from build123d import *

# Parameters (mm, degrees)
PAD048_DEPTH    = 20
PAD049_DEPTH    = 3
CHAMFER030_SIZE = 2
CHAMFER031_SIZE = 1
SKETCH091_R     = 1.6
POCKET029_DEPTH = 5
CHAMFER032_SIZE = 1
SKETCH092_R     = 1.6
POCKET030_DEPTH = 3
CHAMFER033_SIZE = 1
SKETCH093_R     = 1.6
POCKET031_DEPTH = 3.001
CHAMFER034_SIZE = 1


with BuildPart() as part:
    # Sketch089 → Pad048 (new body)
    with BuildSketch(Plane.XY):
        Polygon((19.414214, 3), (8.313708, 3), (3, 8.313708), (3, 19.414214), (1, 21.414214), (0, 21.414214), (0, 1.414214), (1.414214, 0), (21.414214, 0), (21.414214, 1), align=None)
    extrude(amount=-PAD048_DEPTH)

    # Sketch090 → Pad049 (join)
    with BuildSketch(Plane.XY):
        Polygon((0, 21.414214), (20, 21.414214), (21.414214, 20), (21.414214, 0), (1.414214, 0), (0, 1.414214), align=None)
    extrude(amount=PAD049_DEPTH)

    # Chamfer030
    chamfer030_edges = [part.edges().sort_by_distance(p)[0] for p in [
        (21.414214, 10.5, 0),
        (20.707107, 20.707107, 0),
        (10.5, 21.414214, 0),
    ]]
    chamfer(chamfer030_edges, length=CHAMFER030_SIZE)

    # Chamfer031
    chamfer031_edges = [part.edges().sort_by_distance(p)[0] for p in [
        (0.707107, 0.707107, 3),
        (11.414214, 0, 3),
        (0, 11.414214, 3),
    ]]
    chamfer(chamfer031_edges, length=CHAMFER031_SIZE)

    # Sketch091 (on Face15 of Chamfer031) → Pocket029 (cut)
    with BuildSketch(Plane(origin=(0, 0, 0), x_dir=(1, 0, 0), z_dir=(0, 0, -1))):
        with Locations((11.207107, -11.085786)):
            Circle(SKETCH091_R)
    extrude(amount=-POCKET029_DEPTH, mode=Mode.SUBTRACT)

    # Chamfer032
    chamfer032_edges = [part.edges().sort_by_distance(p)[0] for p in [
        (9.607107, 11.085786, 0),
    ]]
    chamfer(chamfer032_edges, length=CHAMFER032_SIZE)

    # Sketch092 (on Face16 of Chamfer032) → Pocket030 (cut)
    with BuildSketch(Plane.YZ.offset(3)):
        with Locations((13.863961, -14.5)):
            Circle(SKETCH092_R)
        with Locations((13.863961, -5.5)):
            Circle(SKETCH092_R)
    extrude(amount=-POCKET030_DEPTH, mode=Mode.SUBTRACT)

    # Chamfer033
    chamfer033_edges = [part.edges().sort_by_distance(p)[0] for p in [
        (3, 12.263961, -14.5),
        (3, 12.263961, -5.5),
    ]]
    chamfer(chamfer033_edges, length=CHAMFER033_SIZE)

    # Sketch093 (on Face9 of Chamfer033) → Pocket031 (cut, through all)
    with BuildSketch(Plane(origin=(0, 3, 0), x_dir=(-1, 0, 0), z_dir=(0, 1, 0))):
        with Locations((-13.863961, -5.5)):
            Circle(SKETCH093_R)
        with Locations((-13.863961, -14.5)):
            Circle(SKETCH093_R)
    extrude(amount=-POCKET031_DEPTH, mode=Mode.SUBTRACT)

    # Chamfer034
    chamfer034_edges = [part.edges().sort_by_distance(p)[0] for p in [
        (15.463961, 3, -5.5),
        (15.463961, 3, -14.5),
    ]]
    chamfer(chamfer034_edges, length=CHAMFER034_SIZE)


with BuildPart() as part_1:
    # Body088 placement: moved
    add(part.part.moved(Location((0, 0, -18))))


solid = part_1.part
For this review, take the finished solid that the model builds, in its own axes (mm). A direction names the side the tool comes from. Coordinates: 2 decimals unless noted, no trailing zeros. Order: outer loops, then holes, each group sorted by start corner. A loop starts at its lowest first (then second) coordinate and runs counter-clockwise, first axis right, second up. Notation, with made-up numbers: (46.25, 86) - (93.25, 86) arc R19 cw to (93.25, 122) - close; hole circle Ø2 at (84, 47). An arc over 180 degrees is marked (long way). Answer as CSV lines item,"result". Start each with the question number.
1) Machinability: for faces 1 (the cylindrical face through (1.01, 14.6, -33.92)), 2 (the flat face through (20.4, 10.633, -17.014)), which of the approach directions +Z, -Z, +X, -X, +Y, -Y give a long, thin tool a straight path to every point of the face, cutting with its end or side? Answer none if there is none.
2) Add section A-A (y = 18.75). State the section outline as (x, z) points, then the cut area to 3 significant figures.
3) Draft analysis for pull direction Z (two halves, no side actions). For faces 3 (the flat face through (20.428, 1.986, -26.846)), 4 (the flat face through (13.1, 13.1, -18)), 5 (the cylindrical face through (1.014, 13.656, -21.914)), state which applies: +Z half, -Z half, draft (parallel to the pull), parting line (faces both ways), or undercut.
4) Insertion check: P1, Ø5, axis at y = 13.86, z = -32.5, coming from the +X side; P2, Ø6, axis at x = 19, y = 16, coming from the -Z side; P3, Ø5, axis at x = 11.21, y = 11.09, coming from the -Z side; P4, Ø3, axis at x = 13.86, z = -32.5, coming from the -Y side. Each pin has a flat end and moves straight along its axis. Give the tip position at first contact, or say it passes through.
5) To check wall thickness, follow line 1 along Z through (x, y) = (15.25, 10); line 2 along Y through (x, z) = (18, -23.75). State the ranges of each line that lie inside material, in increasing order. Write a range as [from, to].
6) Add section D-D (z = -29.5). State the section outline as (x, y) points.
7) Add section C-C (z = -32.5). State the section outline as (x, y) points.
Result:
1,face 1,"+X, -X"
1,face 2,"-Z, +X, +Y"
2,outline,"(0, -38) - (3, -38) - (3, -18) - (19.41, -18) - (21.41, -16) - (21.41, -15) - (1, -15) - (0, -16) - close"
2,area,"122 mm^2"
3,face 3,"draft"
3,face 4,"-Z half"
3,face 5,"undercut"
4,P1,"x = 2.9"
4,P2,"z = -18"
4,P3,"z = -17.91"
4,P4,"through"
5,line 1,"[-18, -15]"
5,line 2,"[0, 3]"
6,outline,"(0, 1.41) - (1.41, 0) - (21.41, 0) - (21.41, 1) - (19.41, 3) - (8.31, 3) - (3, 8.31) - (3, 19.41) - (1, 21.41) - (0, 21.41) - close"
7,outline,"(0, 1.41) - (1.41, 0) - (12.26, 0) - (12.26, 2) - (11.26, 3) - (8.31, 3) - (3, 8.31) - (3, 11.26) - (2, 12.26) - (0, 12.26) - close; (0, 15.46) - (2, 15.46) - (3, 16.46) - (3, 19.41) - (1, 21.41) - (0, 21.41) - close; (15.46, 0) - (21.41, 0) - (21.41, 1) - (19.41, 3) - (16.46, 3) - (15.46, 2) - close"
